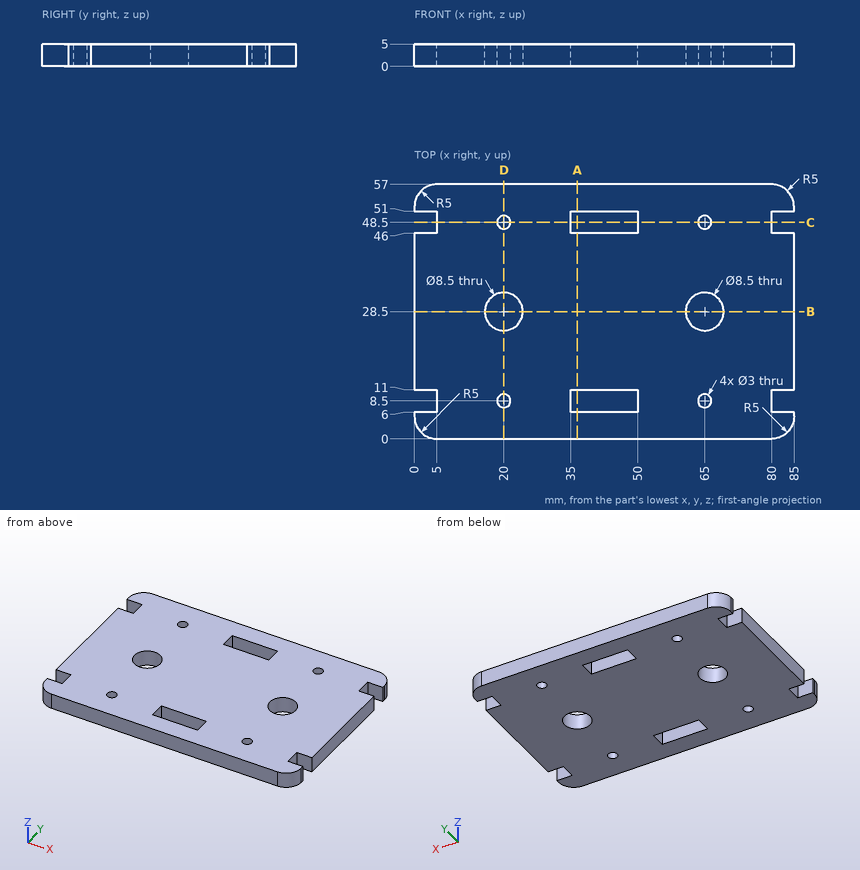
Input: dimensioned drawing with shaded views. Units: mm. Origin: part minimum x, y, z. Coordinates: 2 decimals unless noted, no trailing zeros. Loops run counter-clockwise (first coordinate to the right, second up) from the corner with the lowest first, then second, coordinate; pieces in that order, holes last. Notation, with made-up numbers: M 26.25,39 L 67.25,39 A13 cw 67.25,63 Z; hole C 28.25,72.25 d1. An arc over 180 degrees is marked long. One line per item, written item: value.
(1) Section D-D (x = 20). Output: boundary loops of the cut face in (y, z).
Filled in:
outline: M 0,0 L 7,0 L 7,5 L 0,5 Z; M 10,0 L 24.25,0 L 24.25,5 L 10,5 Z; M 32.75,0 L 47,0 L 47,5 L 32.75,5 Z; M 50,0 L 57,0 L 57,5 L 50,5 Z
(2) Line query: line 1 along Y through (x, z) = (20, 1.55); line 2 along Y through (x, z) = (49, 3.5); line 3 along Y through (x, z) = (62.5, 3.75). Output: solid intervals per line, ascending. Write a range as from..to.
Filled in:
line 1: 0..7, 10..24.25, 32.75..47, 50..57
line 2: 0..6, 11..46, 51..57
line 3: 0..25.06, 31.94..57
(3) Pin query (flat end, axial travel): pin 1 (2.5 mm diameter, centred on x = 83, z = 1.5, fed in from +Y); pin 2 (1.5 mm diameter, centred on y = 7.5, z = 1.5, fed in from -X); pin 3 (1.5 mm diameter, centred on y = 7.5, z = 3, fed in from +X). Return the tip coordinate at first contact, or that it passes through.
Filled in:
pin 1: y = 56.68
pin 2: x = 5
pin 3: x = 80
(4) Section A-A (x = 36.5). Output: boundary loops of the cut face in (y, z).
Filled in:
outline: M 0,0 L 6,0 L 6,5 L 0,5 Z; M 11,0 L 46,0 L 46,5 L 11,5 Z; M 51,0 L 57,0 L 57,5 L 51,5 Z
(5) Section C-C (y = 48.5). Output: boundary loops of the cut face in (x, z), and give its area (3 significant figures).
Filled in:
outline: M 5,0 L 18.5,0 L 18.5,5 L 5,5 Z; M 21.5,0 L 35,0 L 35,5 L 21.5,5 Z; M 50,0 L 63.5,0 L 63.5,5 L 50,5 Z; M 66.5,0 L 80,0 L 80,5 L 66.5,5 Z
area: 270 mm^2
(6) Section B-B (y = 28.5). Output: boundary loops of the cut face in (x, z), and give its area (3 significant figures).
Filled in:
outline: M 0,0 L 15.75,0 L 15.75,5 L 0,5 Z; M 24.25,0 L 60.75,0 L 60.75,5 L 24.25,5 Z; M 69.25,0 L 85,0 L 85,5 L 69.25,5 Z
area: 340 mm^2
